Could you check a few things on this model? Use its own coordinates, in mm. Face numbers are marked on the shaded views. A direction names the side the tool comes from. Round coordinates to 2 decimals unless told otherwise and drop trailing zeros. Loops run counter-clockwise (first coordinate to the right, second up) from the corner with the lowest first, then second, coordinate; pieces in that order, holes last. Notation, with made-up numbers: (18.25, 3) - (47.25, 3) arc R37 cw to (47.25, 42) - close; hole circle Ø9 at (29, -3.5). An arc over 180 degrees is marked (long way). Answer as CSV lines item,"result". Start each with the question number.
1) Which directions (+Z, -Z, +X, -X, +Y, -Y) give clear straight access to the entire face, cutting with the end or side of a thin tool? Please do the marked faces 1 and 2.
2) I'm going to push flat-ended pins straight in: pin 1 Ø1.4 at (x, y) = (112, 32.5) entering from -Z; pin 2 Ø8 at (y, z) = (6, -32) entering from -X (3 decimals); pin 3 Ø4.5 at (x, z) = (80.5, -41) entering from +Y; pin 4 Ø8 at (y, z) = (30, -30) entering from -X. Where does each tip first touch, or does it pass through?
3) Suppose I cut it at D-D, the plane x = 66.5. Write out the boundary of the cut face in (y, z).
4) We'd pull the mould along X, two halves only. Please class the marked faces 3 and 4: pulls with the +X half, pulls with the -X half, needs draft (parallel to the pull), parting line crosses it, or undercut.
5) Suppose I cut it at A-A, the plane y = 18. Write out the boundary of the cut face in (x, z), then the cut area to 3 significant figures.
6) Suppose I cut it at B-B, the plane z = -6.01. Write out the boundary of the cut face in (x, y).
7) Please list where these lines run through material, in increasing order: line 1 along Y through (x, z) = (96.5, -45); line 2 along X through (y, z) = (27, -6.5); line 3 along Y through (x, z) = (40, -13).
8) Suppose I cut it at C-C, the plane z = -41. Write out the boundary of the cut face in (x, y).
```python
from build123d import *

# Parameters (mm, degrees)
BOSS_EXTRUDE1_DEPTH = 3.5
FILLET1_SIZE        = 3
SKETCH4_W           = 4.33
SKETCH4_H           = 10
BOSS_EXTRUDE2_DEPTH = 35
SKETCH5_W           = 10
SKETCH5_H           = 5
SKETCH5_R           = 1.55
SKETCH5_W_2         = 4.658740085
SKETCH5_H_2         = 12
BOSS_EXTRUDE3_DEPTH = 4
FILLET2_SIZE        = 1
CUT_EXTRUDE1_DEPTH  = 14
BOSS_EXTRUDE4_DEPTH = 35
SKETCH9_W           = 28
SKETCH9_H           = 14.5
CUT_EXTRUDE2_DEPTH  = 117
SKETCH10_R          = 1.75
CUT_EXTRUDE3_DEPTH  = 117
FILLET3_SIZE        = 4
SKETCH11_R          = 1.55
CUT_EXTRUDE4_DEPTH  = 95
SKETCH12_R          = 1.55
BOSS_EXTRUDE5_DEPTH = 5


with BuildPart() as part:
    # Sketch1 → Boss-Extrude1 (new body)
    with BuildSketch(Plane(origin=(0, 0, 0), x_dir=(1, 0, 0), z_dir=(0, 1, 0))):
        Polygon((35.5, 70), (35.5, 46.99950249), (74.5, 46.99950249), (74.5, 70), (110, 70), (110, 0), (0, 0), (0, 70), align=None)
    extrude(amount=BOSS_EXTRUDE1_DEPTH)

    # Fillet1
    fillet1_edges = [part.edges().sort_by_distance(p)[0] for p in [
        (35.5, 1.75, -46.99950249),
        (74.5, 1.75, -46.99950249),
    ]]
    chamfer(fillet1_edges, length=FILLET1_SIZE)

    # Sketch4 → Boss-Extrude2 (add)
    with BuildSketch(Plane(origin=(0, 3.5, 0), x_dir=(1, 0, 0), z_dir=(0, 1, 0))):
        with Locations((107.835, 5)):
            Rectangle(SKETCH4_W, SKETCH4_H)
        with Locations((2.165, 5)):
            Rectangle(SKETCH4_W, SKETCH4_H)
    extrude(amount=BOSS_EXTRUDE2_DEPTH)

    # Sketch5 → Boss-Extrude3 (add)
    # profile 1 of 6: a face of its own
    with BuildSketch(Plane.XY):
        with Locations((35.6, 6)):
            Rectangle(SKETCH5_W, SKETCH5_H)
        with Locations((35.6, 6)):
            Circle(SKETCH5_R, mode=Mode.SUBTRACT)
    # profile 2 of 6: a face of its own
    with BuildSketch(Plane.XY):
        with Locations((-2.329370043, 32.5)):
            Rectangle(SKETCH5_W_2, SKETCH5_H_2)
        with Locations((-2.329370042, 32.5)):
            Circle(SKETCH5_R, mode=Mode.SUBTRACT)
    # profile 3 of 6: a face of its own
    with BuildSketch(Plane.XY):
        with Locations((-2.329370043, 6)):
            Rectangle(SKETCH5_W_2, SKETCH5_H_2)
        with Locations((-2.329370042, 6)):
            Circle(SKETCH5_R, mode=Mode.SUBTRACT)
    # profile 4 of 6: a face of its own
    with BuildSketch(Plane.XY):
        with Locations((74.4, 6)):
            Rectangle(SKETCH5_W, SKETCH5_H)
        with Locations(Location((74.4, 6, 0), (0, 0, 180))):
            Circle(SKETCH5_R, mode=Mode.SUBTRACT)
    # profile 5 of 6: a face of its own
    with BuildSketch(Plane.XY):
        with Locations((112.329370043, 6)):
            Rectangle(SKETCH5_W_2, SKETCH5_H_2)
        with Locations(Location((112.329370042, 6, 0), (0, 0, 180))):
            Circle(SKETCH5_R, mode=Mode.SUBTRACT)
    # profile 6 of 6: a face of its own
    with BuildSketch(Plane.XY):
        with Locations((112.329370043, 32.5)):
            Rectangle(SKETCH5_W_2, SKETCH5_H_2)
        with Locations(Location((112.329370042, 32.5, 0), (0, 0, 180))):
            Circle(SKETCH5_R, mode=Mode.SUBTRACT)
    extrude(amount=-BOSS_EXTRUDE3_DEPTH)

    # Fillet2
    fillet2_edges = [part.edges().sort_by_distance(p)[0] for p in [
        (69.4, 8.5, -2),
        (79.4, 8.5, -2),
        (114.658740085, 12, -2),
        (114.658740085, 0, -2),
        (114.658740085, 38.5, -2),
        (114.658740085, 26.5, -2),
        (40.6, 8.5, -2),
        (30.6, 8.5, -2),
        (-4.658740085, 26.5, -2),
        (-4.658740085, 38.5, -2),
        (-4.658740085, 0, -2),
        (-4.658740085, 12, -2),
    ]]
    chamfer(fillet2_edges, length=FILLET2_SIZE)

    # Sketch6 → Cut-Extrude1 (cut)
    with BuildSketch(Plane(origin=(0, 3.5, 0), x_dir=(1, 0, 0), z_dir=(0, 1, 0))):
        Polygon((0, 10), (17.75, 70), (0, 70), align=None)
        Polygon((110, 70), (92.25, 70), (110, 10), align=None)
    extrude(amount=-CUT_EXTRUDE1_DEPTH, mode=Mode.SUBTRACT)

    # Sketch8 → Boss-Extrude4 (add)
    with BuildSketch(Plane(origin=(0, 3.5, 0), x_dir=(1, 0, 0), z_dir=(0, 1, 0))):
        Polygon((0, 10), (14.2, 58), (18.53, 58), (4.33, 10), align=None)
        Polygon((91.47, 58), (105.67, 10), (110, 10), (95.8, 58), align=None)
    extrude(amount=BOSS_EXTRUDE4_DEPTH)

    # Sketch9 → Cut-Extrude2 (cut)
    with BuildSketch(Plane.ZY):
        with Locations((-34, 21.25)):
            Rectangle(SKETCH9_W, SKETCH9_H)
    extrude(amount=-CUT_EXTRUDE2_DEPTH, mode=Mode.SUBTRACT)

    # Sketch10 → Cut-Extrude3 (cut)
    with BuildSketch(Plane(origin=(0, 3.5, 0), x_dir=(1, 0, 0), z_dir=(0, 1, 0))):
        with Locations(Location((80.5, 62.75, 0), (0, 0, 270))):
            Circle(SKETCH10_R)
        with Locations(Location((80.5, 41, 0), (0, 0, 270))):
            Circle(SKETCH10_R)
        with Locations(Location((29.5, 41, 0), (0, 0, 90))):
            Circle(SKETCH10_R)
        with Locations(Location((29.5, 62.75, 0), (0, 0, 90))):
            Circle(SKETCH10_R)
    extrude(amount=-CUT_EXTRUDE3_DEPTH, mode=Mode.SUBTRACT)

    # Fillet3
    fillet3_edges = [part.edges().sort_by_distance(p)[0] for p in [
        (11.43, 3.5, -34),
        (98.57, 3.5, -34),
        (4.33, 3.5, -5),
        (105.67, 3.5, -5),
    ]]
    chamfer(fillet3_edges, length=FILLET3_SIZE)

    # Sketch11 → Cut-Extrude4 (cut)
    with BuildSketch(Plane(origin=(0, 38.5, 0), x_dir=(1, 0, 0), z_dir=(0, 1, 0))):
        with Locations(Location((88, 6.01, 0), (0, 0, 270))):
            Circle(SKETCH11_R)
        with Locations(Location((22, 6.01, 0), (0, 0, 270))):
            Circle(SKETCH11_R)
    extrude(amount=-CUT_EXTRUDE4_DEPTH, mode=Mode.SUBTRACT)

    # Sketch12 → Boss-Extrude5 (add)
    # profile 1 of 4: a face of its own
    with BuildSketch(Plane(origin=(0, 38.5, 0), x_dir=(1, 0, 0), z_dir=(0, 1, 0))):
        Polygon((14.2, 58), (9.7, 58), (6.86319811, 48.410810512), (10.45001483, 45.323993792), (11.36319811, 48.410810512), align=None)
        with Locations(Location((10.350531543, 52.593346062, 0), (0, 0, 270))):
            Circle(SKETCH12_R, mode=Mode.SUBTRACT)
    # profile 2 of 4: a face of its own
    with BuildSketch(Plane(origin=(0, 38.5, 0), x_dir=(1, 0, 0), z_dir=(0, 1, 0))):
        Polygon((3.75018599, 22.676685036), (0.9133841, 13.087495548), (0, 10), (-3.472442888, 13.473432491), (-0.74981401, 22.676685036), align=None)
        with Locations(Location((-0.042195961, 17.462999569, 0), (0, 0, 270))):
            Circle(SKETCH12_R, mode=Mode.SUBTRACT)
    # profile 3 of 4: a face of its own
    with BuildSketch(Plane(origin=(0, 38.5, 0), x_dir=(1, 0, 0), z_dir=(0, 1, 0))):
        Polygon((110.74981401, 22.676685036), (106.24981401, 22.676685036), (109.0866159, 13.087495548), (110, 10), (113.472442888, 13.473432491), align=None)
        with Locations(Location((110.042195961, 17.462999569, 0), (0, 0, 90))):
            Circle(SKETCH12_R, mode=Mode.SUBTRACT)
    # profile 4 of 4: a face of its own
    with BuildSketch(Plane(origin=(0, 38.5, 0), x_dir=(1, 0, 0), z_dir=(0, 1, 0))):
        Polygon((103.13680189, 48.410810512), (99.54998517, 45.323993792), (98.63680189, 48.410810512), (95.8, 58), (100.3, 58), align=None)
        with Locations(Location((99.649468457, 52.593346062, 0), (0, 0, 90))):
            Circle(SKETCH12_R, mode=Mode.SUBTRACT)
    extrude(amount=-BOSS_EXTRUDE5_DEPTH)


solid = part.part
```
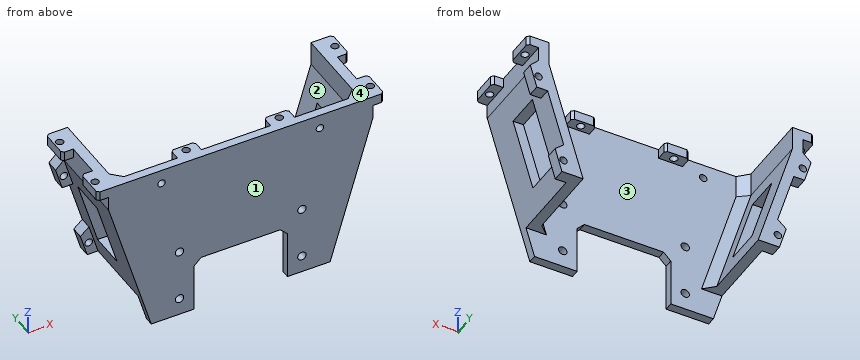
Filled sheet:
1,face 1,"+Z, -Z, +X, -X, -Y"
1,face 2,"+Z, +Y"
2,pin 1,"through"
2,pin 2,"x = 5.325"
2,pin 3,"y = 3.5"
2,pin 4,"x = 4.73"
3,outline,"(0, -47) - (3.5, -47) - (3.5, 0) - (0, 0) - close"
4,face 3,"undercut"
4,face 4,"needs draft"
5,outline,"(0, -10) - (2.96, -20) - (7.29, -20) - (4.33, -10) - (4.33, 0) - (0, 0) - close; (11.24, -48) - (14.2, -58) - (18.53, -58) - (15.57, -48) - close; (91.47, -58) - (95.8, -58) - (98.76, -48) - (94.43, -48) - close; (102.71, -20) - (107.04, -20) - (110, -10) - (110, 0) - (105.67, 0) - (105.67, -10) - close"
5,area,"260 mm²"
6,outline,"(0, 0) - (20.45, 0) - (20.45, 3.5) - (8.33, 3.5) - (4.33, 7.5) - (4.33, 38.5) - (0, 38.5) - close; (23.55, 0) - (86.45, 0) - (86.45, 3.5) - (23.55, 3.5) - close; (89.55, 0) - (110, 0) - (110, 38.5) - (105.67, 38.5) - (105.67, 7.5) - (101.67, 3.5) - (89.55, 3.5) - close"
7,line 1,"0 to 14, 28.5 to 38.5"
7,line 2,"0 to 4.33, 105.67 to 110"
7,line 3,"0 to 3.5"
8,outline,"(9.17, 0) - (27.75, 0) - (27.75, 3.5) - (17.67, 3.5) - (13.5, 7.5) - (13.5, 14) - (9.17, 14) - close; (9.17, 28.5) - (13.5, 28.5) - (13.5, 38.5) - (9.17, 38.5) - close; (31.25, 0) - (78.75, 0) - (78.75, 3.5) - (31.25, 3.5) - close; (82.25, 0) - (100.83, 0) - (100.83, 14) - (96.5, 14) - (96.5, 7.5) - (92.33, 3.5) - (82.25, 3.5) - close; (96.5, 28.5) - (100.83, 28.5) - (100.83, 38.5) - (96.5, 38.5) - close"
